Autodesk Fusion 360 part; units mm, degrees
sketch "Front" plane through (0, 0, 0) normal (0, 1, 0) x (1, 0, 0)
  line L0 (415, -143.75) -> (-415, -143.75)
  line L1 (-415, -143.75) -> (-415, 143.75)
  line L2 (-415, 143.75) -> (415, 143.75)
  line L3 (415, 143.75) -> (415, -143.75)
  line L4 (415, -143.75) -> (-415, 143.75) construction
  line L5 (-415, -143.75) -> (415, 143.75) construction
  line L6 (-400, -101.125) -> (400, -101.125) construction
  line L7 (-400, -71.125) -> (400, -71.125) construction
  line L8 (-400, 93.875) -> (400, 93.875) construction
  line L9 (-400, 123.875) -> (400, 123.875) construction
  line L10 (-335, -110) -> (-335, 130) construction
  line L11 (-185, -110) -> (-185, 130) construction
  line L12 (-35, -110) -> (-35, 130) construction
  line L13 (115, -110) -> (115, 130) construction
  line L14 (265, -110) -> (265, 130) construction
  circle A0 centre (-335, -101.125) radius 3
  circle A1 centre (-335, -71.125) radius 3
  circle A2 centre (-335, 93.875) radius 3
  circle A3 centre (-335, 123.875) radius 3
  circle A4 centre (-185, 123.875) radius 3
  circle A5 centre (-185, 93.875) radius 3
  circle A6 centre (-185, -71.125) radius 3
  circle A7 centre (-185, -101.125) radius 3
  circle A8 centre (-35, -101.125) radius 3
  circle A9 centre (-35, -71.125) radius 3
  circle A10 centre (-35, 93.875) radius 3
  circle A11 centre (-35, 123.875) radius 3
  circle A12 centre (115, -101.125) radius 3
  circle A13 centre (115, -71.125) radius 3
  circle A14 centre (115, 93.875) radius 3
  circle A15 centre (115, 123.875) radius 3
  circle A16 centre (265, 123.875) radius 3
  circle A17 centre (265, 93.875) radius 3
  circle A18 centre (265, -71.125) radius 3
  circle A19 centre (265, -101.125) radius 3
  line L15 (-400, -120) -> (-400, 130) construction
  line L16 (345, -110) -> (345, 130) construction
  line L17 (-360, 49.875) -> (300, 49.875) construction
  line L18 (-360, 3.875) -> (300, 3.875) construction
  line L19 (-332, -10) -> (-332, 60) construction
  line L20 (263, -10) -> (263, 60) construction
  line L21 (276, -10) -> (276, 60) construction
  circle A20 centre (-332, 3.875) radius 3.5
  circle A21 centre (-332, 49.875) radius 3.5
  circle A22 centre (263, 3.875) radius 3.5
  circle A23 centre (276, 3.875) radius 3.5
  circle A24 centre (263, 49.875) radius 3.5
  circle A25 centre (276, 49.875) radius 3.5
  circle A26 centre (-400, -55) radius 4
  circle A27 centre (-400, 65) radius 4
  circle A28 centre (345, 114.875) radius 4
  circle A29 centre (345, -85.125) radius 4
  line L22 (415, -9.625) -> (322.5, -9.625)
  line L23 (322.5, -9.625) -> (322.5, 63.375)
  line L24 (322.5, 63.375) -> (415, 63.375)
  line L25 (415, 63.375) -> (415, -9.625)
  line L26 (384.5, -50) -> (384.5, 85) construction
  line L27 (360.5, -50) -> (360.5, 85) construction
  line L28 (355, -18.125) -> (390, -18.125) construction
  line L29 (350, 6.875) -> (390, 6.875) construction
  line L30 (350, 46.875) -> (390, 46.875) construction
  line L31 (350, 71.875) -> (390, 71.875) construction
  circle A30 centre (360.5, -18.125) radius 3
  circle A31 centre (384.5, -18.125) radius 3
  circle A32 centre (360.5, 71.875) radius 3
  circle A33 centre (384.5, 71.875) radius 3
  circle A34 centre (360.5, 46.875) radius 2.5
  circle A35 centre (384.5, 46.875) radius 2.5
  circle A36 centre (360.5, 6.875) radius 2.5
  circle A37 centre (384.5, 6.875) radius 2.5
  dimension "d1" = 830
  dimension "d2" = 287.5
  dimension "d3" = 30
  dimension "d4" = 30
  dimension "d5" = 165
  dimension "d6" = 19.875
  dimension "d7" = 150
  dimension "d8" = 150
  dimension "d9" = 150
  dimension "d10" = 150
  dimension "d11" = 80
  dimension "d12" = 6
  dimension "d13" = 6
  dimension "d14" = 6
  dimension "d15" = 6
  dimension "d16" = 6
  dimension "d17" = 6
  dimension "d18" = 6
  dimension "d19" = 6
  dimension "d20" = 6
  dimension "d21" = 6
  dimension "d22" = 6
  dimension "d23" = 6
  dimension "d24" = 6
  dimension "d25" = 6
  dimension "d26" = 6
  dimension "d27" = 6
  dimension "d28" = 6
  dimension "d29" = 6
  dimension "d30" = 6
  dimension "d31" = 6
  dimension "d32" = 15
  dimension "d33" = 70
  dimension "d34" = 46
  dimension "d36" = 75
  dimension "d37" = 83
  dimension "d38" = 13
  dimension "d39" = 595
  dimension "d40" = 7
  dimension "d41" = 7
  dimension "d42" = 7
  dimension "d43" = 7
  dimension "d44" = 7
  dimension "d45" = 7
  dimension "d46" = 8
  dimension "d47" = 8
  dimension "d48" = 120
  dimension "d49" = 78.75
  dimension "d50" = 8
  dimension "d51" = 8
  dimension "d52" = 200
  dimension "d54" = 16
  dimension "d55" = 745
  dimension "d56" = 92.5
  dimension "d57" = 73
  dimension "d58" = 13.5
  dimension "d59" = 24
  dimension "d60" = 30.5
  dimension "d61" = 25
  dimension "d62" = 25
  dimension "d63" = 40
  dimension "d64" = 16.5
  dimension "d65" = 6
  dimension "d66" = 6
  dimension "d67" = 6
  dimension "d68" = 6
  dimension "d69" = 5
  dimension "d70" = 5
  dimension "d71" = 5
  dimension "d72" = 5
extrude "Extrude1" add sketch "Front" against normal blind 4 contours L3 L22 L23 L24 L25
extrude "Extrude2" add sketch "Front" against normal blind 18 contours L0 L1 L2 L3 L22 L23 L24
fillet "Fillet1" radius 6.35 2 edges at (322.5, -11, -63.375) (322.5, -11, 9.625)
Verification items for the finished model (mm, model axes). A direction names the side the tool comes from. Give positions to 0.01 mm unless a question says otherwise; leave off trailing zeros. Write each loop counter-clockwise with the first axis right and the second up, starting at its lowest first coordinate (ties: lowest second). Pieces come first, ordered by that corner, then holes.
(1) Cross-section at A-A (z = -27.5). Enter the section's corners in (x, y), plus the area to 3 significant figures.
(2) Material ranges on line 1 (Z direction, x = 276, y = -7.5) (3 decimals); line 2 (X direction, y = -15, z = -114); line 3 (Z direction, x = 360.5, y = -2.05) (3 decimals), recorded low to high.
(3) Cross-section at B-B (y = -10). State how many separate pieces and enclosed holes the cut face has, plus the area to 3 significant figures.
(4) Mould release check, pull along Z, two halves, no side actions. Record for faces 1 (the face through (-6, -9, -143.75)), 2 (the face through (373, -11, 9.625)), 3 (the face through (-415, -9, 2)): +Z half, -Z half, draft (parallel to the pull), parting line (faces both ways), or undercut.
(5) Gauge pin test, flat ends, axial feed: pin 1 (3.5 mm diameter, centred on x = -35, z = 71.125, fed in from +Y); pin 2 (3 mm diameter, centred on y = -6, z = -30.5, fed in from +X); pin 3 (6.5 mm diameter, centred on x = 384.5, z = -46.875, fed in from -Y). Record the tip position at first contact, or that the pin passes through.
(6) Access from +Z, -Z, +X, -X, +Y, -Y to the whole of each face (thin tool, end or side, straight path). Record for faces 4 (the face through (371, -11, -63.375)), 5 (the face through (415, -3, -2)).
Worked out:
1. outline: (-415, -18) - (322.5, -18) - (322.5, -4) - (415, -4) - (415, 0) - (-415, 0) - close
1. area: 13,600 mm2
2. line 1: z = -143.75 to -53.375, -46.375 to -7.375, -0.375 to 143.75
2. line 2: x = -415 to 341.1, 348.9 to 415
2. line 3: z = -143.75 to -74.875, -68.875 to -49.375, -44.375 to -9.375, -4.375 to 15.125, 21.125 to 143.75
3. separate pieces: 1
3. enclosed holes: 34
3. area: 231,000 mm2
4. face 1: -Z half
4. face 2: undercut
4. face 3: draft
5. pin 1: passes through
5. pin 2: stops at x = 322.5
5. pin 3: stops at y = -4
6. face 4: +X, -Y
6. face 5: +Z, -Z, +X, +Y, -Y
